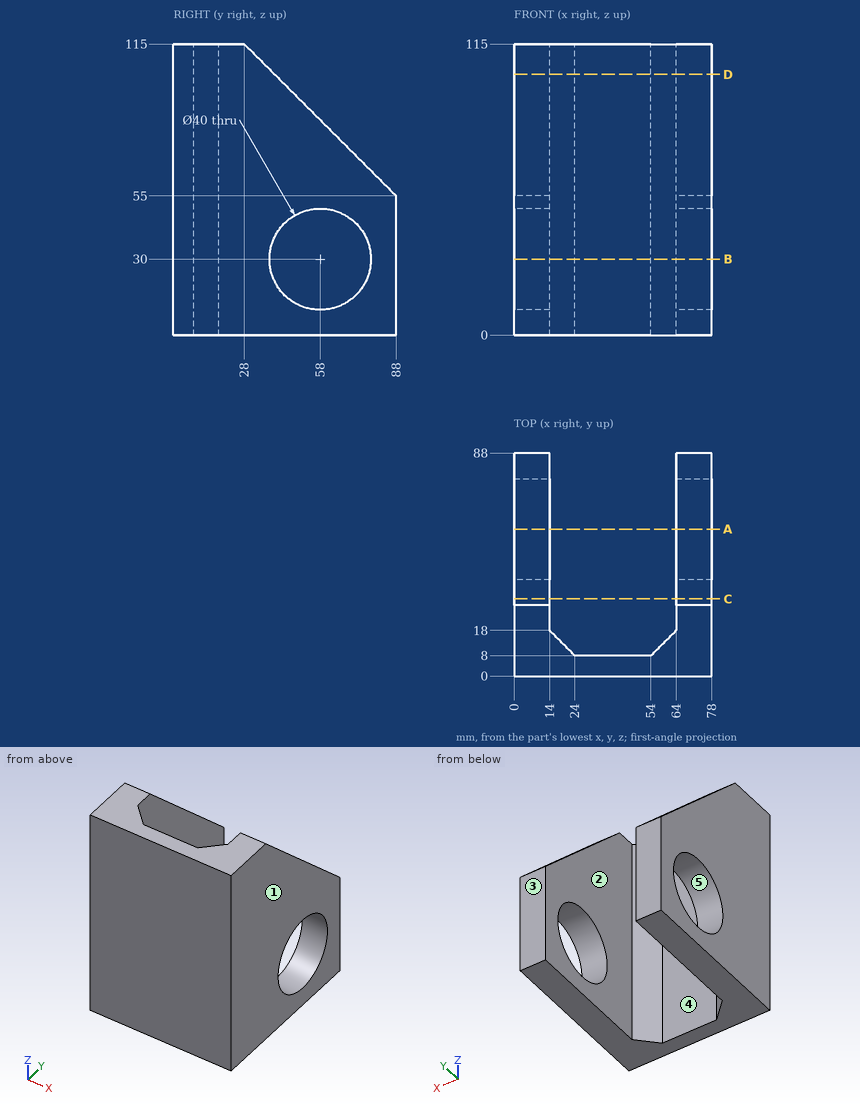
Here's the drawing with two shaded views (mm, measured from the low corner). I have some questions. A direction names the side the tool comes from. Round coordinates to 2 decimals unless told otherwise and drop trailing zeros. Loops run counter-clockwise (first coordinate to the right, second up) from the corner with the lowest first, then second, coordinate; pieces in that order, holes last. Notation, with made-up numbers: M 16.5,49.25 L 67.5,49.25 A5 cw 67.5,53.25 Z; hole C 86.25,8.5 d4. An arc over 180 degrees is marked long. Put each result on its own line as item: value.
Q1. Thinking about a two-plate mould opening in X: for the marked faces 1, 2 and 3, which applies, released by +X, released by -X, zero draft, split by the parting line, or undercut?
Check result:
face 1: released by +X
face 2: undercut
face 3: zero draft
Q2. I need wall thicknesses on probe 1 along X at (y, z) = (39.5, 53); probe 2 along Y at (x, z) = (74, 30); probe 3 along Y at (x, z) = (40, 56.5). Which ranges of each line are inside material? Lowest first, please.
Check result:
probe 1: 0 to 14, 64 to 78
probe 2: 0 to 38, 78 to 88
probe 3: 0 to 8
Q3. On a 3-axis mill with a long thin cutter (end or side, diameter ignored), from which of +Z, -Z, +X, -X, +Y, -Y can I reach the whole of each face in a straight line? I mean the marked faces 4 and 5. Say none if no direction works.
Check result:
face 4: +Z, -Z, +Y
face 5: +X, -X
Q4. Imagine slicing it at A-A (y = 58). Write out the boundary of the cut face in (x, z), then the cut area to 3 significant figures.
Check result:
outline: M 0,0 L 14,0 L 14,10 L 0,10 Z; M 0,50 L 14,50 L 14,85 L 0,85 Z; M 64,0 L 78,0 L 78,10 L 64,10 Z; M 64,50 L 78,50 L 78,85 L 64,85 Z
area: 1,260 mm2
Q5. Imagine slicing it at D-D (z = 103). Write out the boundary of the cut face in (x, y).
Check result:
outline: M 0,0 L 78,0 L 78,40 L 64,40 L 64,18 L 54,8 L 24,8 L 14,18 L 14,40 L 0,40 Z
Q6. Imagine slicing it at B-B (z = 30). Write out the boundary of the cut face in (x, y).
Check result:
outline: M 0,0 L 78,0 L 78,38 L 64,38 L 64,18 L 54,8 L 24,8 L 14,18 L 14,38 L 0,38 Z; M 0,78 L 14,78 L 14,88 L 0,88 Z; M 64,78 L 78,78 L 78,88 L 64,88 Z
Q7. Imagine slicing it at C-C (y = 30.5). Write out the boundary of the cut face in (x, z), then the cut area to 3 significant figures.
Check result:
outline: M 0,0 L 14,0 L 14,112.5 L 0,112.5 Z; M 64,0 L 78,0 L 78,112.5 L 64,112.5 Z
area: 3,150 mm2
Q8. For pin 1 (4 mm diameter, centred on x = 66.5, y = 58, fed in from +Z); pin 2 (9 mm diameter, centred on x = 44, z = 75, fed in from +Y), each with a flat end and sliding along its axis, tell me the tip position at first contact or that it passes through.
Check result:
pin 1: z = 87
pin 2: y = 8
